from build123d import *

# Parameters (mm, degrees)
BOSS_EXTRUDE1_DEPTH = 15.3
SKETCH3_R           = 4.75
BOSS_EXTRUDE2_DEPTH = 9
CUT_EXTRUDE1_DEPTH  = 1.5


with BuildPart() as part:
    # Sketch2 → Boss-Extrude1 (new body)
    with BuildSketch(Plane.XY):
        with BuildLine():
            Line((-20, 9), (-20, -41))
            Line((-20, -41), (20, -41))
            Line((20, -41), (20, 9))
            Line((20, 9), (6.25, 9))
            Line((6.25, 9), (6.25, 0))
            ThreePointArc((6.25, 0), (0, -6.25), (-6.25, 0))
            Line((-6.25, 0), (-6.25, 9))
            Line((-6.25, 9), (-20, 9))
        make_face()
    extrude(amount=-BOSS_EXTRUDE1_DEPTH)

    # Sketch3 → Boss-Extrude2 (add)
    with BuildSketch(Plane(origin=(0, 0, -15.3), x_dir=(-1, 0, 0), z_dir=(0, 0, -1))):
        with BuildLine():
            Line((6.25, 0), (6.25, 9))
            Line((6.25, 9), (-6.25, 9))
            Line((-6.25, 9), (-6.25, 0))
            ThreePointArc((-6.25, 0), (0, -6.25), (6.25, 0))
        make_face()
        Circle(SKETCH3_R, mode=Mode.SUBTRACT)
    extrude(amount=-BOSS_EXTRUDE2_DEPTH)

    # Sketch4 → Cut-Extrude1 (cut)
    with BuildSketch(Plane.XY.offset(-6.3)):
        with BuildLine():
            Line((-9, 0), (-9, 9))
            ThreePointArc((-9, 9), (0, 18), (9, 9))
            Line((9, 9), (9, 0))
            ThreePointArc((9, 0), (0, -9), (-9, 0))
        make_face()
    extrude(amount=-CUT_EXTRUDE1_DEPTH, mode=Mode.SUBTRACT)


solid = part.part
Check sheet for the modelled part. Datum: model origin and axes. Units: mm. A direction names the side the tool comes from. Round coordinates to 2 decimals unless told otherwise and drop trailing zeros. Order: outer loops, then holes, each group sorted by start corner. A loop starts at its lowest first (then second) coordinate and runs counter-clockwise, first axis right, second up.
Q1. Cross-section at B-B, the plane y = 3.5. Enter the section's corners in (x, z), plus the area to 3 significant figures.
Filled sheet:
outline: (-20, -15.3) - (-3.21, -15.3) - (-3.21, -7.8) - (-9, -7.8) - (-9, -6.3) - (-6.25, -6.3) - (-6.25, 0) - (-20, 0) - close; (3.21, -15.3) - (20, -15.3) - (20, 0) - (6.25, 0) - (6.25, -6.3) - (9, -6.3) - (9, -7.8) - (3.21, -7.8) - close
area: 458 mm2
Q2. Set-up check for faces 1 (the face through (6.25, 5, -3)), 2 (the face through (0, -16, 0)), 3 (the face through (9, 5, -7)): record each of +Z, -Z, +X, -X, +Y, -Y from which the full face is reachable in a straight line by a thin tool's end or side.
Filled sheet:
face 1: +Z, +Y
face 2: +Z, +X, -X, +Y, -Y
face 3: +Y
Q3. Scan lines: L1, parallel to Y at x = 0, z = -13.5; L2, parallel to X at y = 3, z = -6.75; L3, parallel to X at y = -0.5, z = -5. Record each from-to range of solid material in increasing order.
Filled sheet:
L1: y = -41 to -4.75, 4.75 to 9
L2: x = -20 to -9, 9 to 20
L3: x = -20 to -6.23, 6.23 to 20
Q4. Cross-section at A-A, the plane x = 0. Enter the section's corners in (y, z), plus the area to 3 significant figures.
Filled sheet:
outline: (-41, -15.3) - (-4.75, -15.3) - (-4.75, -7.8) - (-9, -7.8) - (-9, -6.3) - (-6.25, -6.3) - (-6.25, 0) - (-41, 0) - close; (4.75, -15.3) - (9, -15.3) - (9, -7.8) - (4.75, -7.8) - close
area: 571 mm2
Q5. Depth check by flat-ended pin: P1, Ø5.5, axis at x = -0.5, y = 1, coming from the -Z side. Enter the tip coordinate at first touch or a pass-through.
Filled sheet:
P1: passes through
Q6. Cross-section at C-C, the plane z = -4.25. Enter the section's corners in (x, y), plus the area to 3 significant figures.
Filled sheet:
outline: (-20, -41) - (20, -41) - (20, 9) - (6.25, 9) - (6.25, 0) arc R6.25 cw to (-6.25, 0) - (-6.25, 9) - (-20, 9) - close
area: 1,830 mm2
Q7. Draft check along Z on faces 4 (the face through (0, 9, -9)), 5 (the face through (1, -7, -6.3)), 6 (the face through (0, -16, -15.3)), 7 (the face through (0, -9, -7)). Enter one of: pulls with the +Z half, pulls with the -Z half, needs draft (parallel to the pull), parting line crosses it, or undercut.
Filled sheet:
face 4: needs draft
face 5: undercut
face 6: pulls with the -Z half
face 7: undercut
